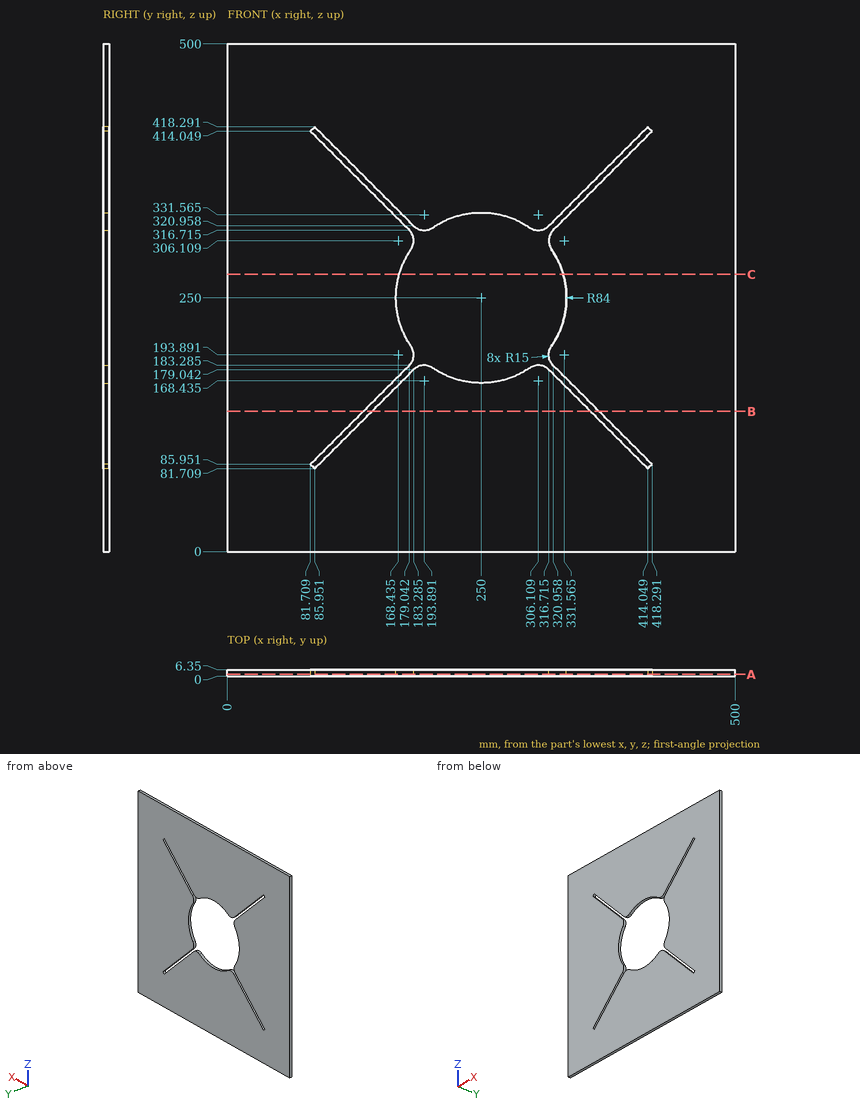
Verification items for this drawing (mm, ordinates from the low corner). Coordinates: 2 decimals unless noted, no trailing zeros. Loops run counter-clockwise (first coordinate to the right, second up) from the corner with the lowest first, then second, coordinate; pieces in that order, holes last. Notation, with made-up numbers: (39, -30.5) -> (76, -30.5) arc R17 cw to (76, -4.5) -> close; hole circle Ø11 at (47.5, 21). An arc over 180 degrees is marked (long way). Answer in a Markdown table with one row per item. Add a question column.
1. Depth check by flat-ended pin: P1, Ø2, axis at y = 2.5, z = 222, coming from the -X side. Enter the tip coordinate at first touch or a pass-through.
2. Section check A-A, the plane y = 1.5. Enter the section's corners in (x, z) (1 decimal), then the cut area to 3 significant figures.
3. Section check C-C, the plane z = 273. Enter the section's corners in (x, y), then the cut area to 3 significant figures.
4. Section check B-B, the plane z = 138. Enter the section's corners in (x, y).
5. Material ranges on probe 1 along Z at (x, y) = (154, 0.75) (1 decimal); probe 2 along Z at (x, y) = (345, 2) (1 decimal); probe 3 along X at (y, z) = (5.25, 321) (1 decimal), recorded low to high. Write a range as [from, to].
Derived:
| question | item | result |
|---|---|---|
| 1 | P1 | stops at x = 0 |
| 2 | outline | (0, 0) -> (500, 0) -> (500, 500) -> (0, 500) -> close; hole (81.7, 86) -> (86, 81.7) -> (183.3, 179) arc R15 cw to (202.4, 180.8) arc R84 ccw to (297.6, 180.8) arc R15 cw to (316.7, 179) -> (414, 81.7) -> (418.3, 86) -> (321, 183.3) arc R15 cw to (319.2, 202.4) arc R84 ccw to (319.2, 297.6) arc R15 cw to (321, 316.7) -> (418.3, 414) -> (414, 418.3) -> (316.7, 321) arc R15 cw to (297.6, 319.2) arc R84 ccw to (202.4, 319.2) arc R15 cw to (183.3, 321) -> (86, 418.3) -> (81.7, 414) -> (179, 316.7) arc R15 cw to (180.8, 297.6) arc R84 ccw to (180.8, 202.4) arc R15 cw to (179, 183.3) -> close |
| 2 | area | 224,000 mm² |
| 3 | outline | (0, 0) -> (169.21, 0) -> (169.21, 6.35) -> (0, 6.35) -> close; (330.79, 0) -> (500, 0) -> (500, 6.35) -> (330.79, 6.35) -> close |
| 3 | area | 2,150 mm² |
| 4 | outline | (0, 0) -> (133.76, 0) -> (133.76, 6.35) -> (0, 6.35) -> close; (142.24, 0) -> (357.76, 0) -> (357.76, 6.35) -> (142.24, 6.35) -> close; (366.24, 0) -> (500, 0) -> (500, 6.35) -> (366.24, 6.35) -> close |
| 5 | probe 1 | z = [0, 149.8], [158.2, 341.8], [350.2, 500] |
| 5 | probe 2 | z = [0, 150.8], [159.2, 340.8], [349.2, 500] |
| 5 | probe 3 | x = [0, 174.8], [183.2, 205.1], [294.9, 316.8], [325.2, 500] |
